```python
from build123d import *

# Parameters (mm, degrees)
SKETCH1_W           = 89
SKETCH1_H           = 57
BOSS_EXTRUDE1_DEPTH = 8
SKETCH2_W           = 32
SKETCH2_H           = 35.5
SKETCH2_H_2         = 6
SKETCH2_W_2         = 19
SKETCH2_H_3         = 1
CUT_EXTRUDE2_DEPTH  = 106.990565618
SKETCH3_R           = 2
CUT_EXTRUDE3_DEPTH  = 6.7


with BuildPart() as part:
    # Sketch1 → Boss-Extrude1 (new body)
    with BuildSketch(Plane(origin=(0, 0, 0), x_dir=(1, 0, 0), z_dir=(0, 1, 0))):
        with Locations((44.5, 28.5)):
            Rectangle(SKETCH1_W, SKETCH1_H)
    extrude(amount=BOSS_EXTRUDE1_DEPTH)

    # Sketch2 → Cut-Extrude2 (cut, through all)
    with BuildSketch(Plane(origin=(0, 8, 0), x_dir=(1, 0, 0), z_dir=(0, 1, 0))):
        with Locations((23.5, 28.25)):
            Rectangle(SKETCH2_W, SKETCH2_H)
        with Locations((23.5, 53)):
            Rectangle(SKETCH2_W, SKETCH2_H_2)
        with Locations((49, 53)):
            Rectangle(SKETCH2_W_2, SKETCH2_H_2)
        with Locations((49, 56.5)):
            Rectangle(SKETCH2_W_2, SKETCH2_H_3)
        with Locations((23.5, 56.5)):
            Rectangle(SKETCH2_W, SKETCH2_H_3)
    extrude(amount=-CUT_EXTRUDE2_DEPTH, mode=Mode.SUBTRACT)

    # Sketch3 → Cut-Extrude3 (cut)
    with BuildSketch(Plane.XY):
        with Locations((3.75, 4)):
            Circle(SKETCH3_R)
        with Locations((79, 4)):
            Circle(SKETCH3_R)
    cut_extrude3 = extrude(amount=-CUT_EXTRUDE3_DEPTH, mode=Mode.SUBTRACT)

    # Mirror1: Cut-Extrude3 across plane
    add(cut_extrude3.mirror(Plane.XY.offset(-28.5)), mode=Mode.SUBTRACT)


solid = part.part
```
The model under review builds one solid part; all positions refer to its coordinate system, in mm. A direction names the side the tool comes from. Round coordinates to 2 decimals unless told otherwise and drop trailing zeros. Loops run counter-clockwise (first coordinate to the right, second up) from the corner with the lowest first, then second, coordinate; pieces in that order, holes last. Notation, with made-up numbers: (70, 77) -> (87, 77) arc R21 ccw to (87, 105) -> close; hole circle Ø5 at (-18.75, 21.5). An arc over 180 degrees is marked (long way). Answer as a JSON object with one key per item and string values. Group by question number.
1) We need section D-D on x = 3.75. Write out the cut boundary in (y, z).
2) We need section B-B on z = -34. Write out the cut boundary in (x, y), then the cut area to 3 significant figures.
3) We need section C-C on y = 7. Write out the cut boundary in (x, z).
4) For line 1 (X direction, y = 4.5, z = -17.5); line 2 (Z direction, x = 13, y = 6.5); line 3 (Y direction, x = 3.75, z = -55.5), list the stretches that pass through material, from the lowest coordinate up. Write a range as [from, to].
5) We need section A-A on x = 32.5. Write out the cut boundary in (y, z).
6) For faces 1 (the face through (7.5, 4, -54)), 2 (the face through (7.5, 4, -28)), 3 (the face through (4, 4, -50.3)), list the 3-axis set-ups (+Z, -Z, +X, -X, +Y, -Y) from which the entire face can be reached by the end or side of a thin tool; tool diameter is ignored.
7) Mouldability with a two-part tool opening along X and no side actions: class faces 4 (the face through (54, 0, -29)), 5 (the face through (80.908, 4.601, -53.697)), 6 (the face through (89, 4, -28)), 7 (the face through (39.5, 4, -28)) as released by +X, released by -X, zero draft, split by the parting line, or undercut.
8) For pin 1 Ø3.5 at (x, y) = (79, 4) entering from -Z; pin 2 Ø2.5 at (x, y) = (43, 2.5) entering from -Z; pin 3 Ø2 at (x, z) = (38, -42) entering from +Y; pin 4 Ø1.2 at (x, y) = (78.5, 5) entering from +Z, all flat-tipped, find the tip position at first contact; note any pin that passes through.
Result set:
{
 "1": {"outline": "(0, -57) -> (2, -57) -> (2, -50.3) -> (6, -50.3) -> (6, -57) -> (8, -57) -> (8, 0) -> (6, 0) -> (6, -6.7) -> (2, -6.7) -> (2, 0) -> (0, 0) -> close"},
 "2": {"outline": "(0, 0) -> (7.5, 0) -> (7.5, 8) -> (0, 8) -> close; (39.5, 0) -> (89, 0) -> (89, 8) -> (39.5, 8) -> close", "area": "456 mm²"},
 "3": {"outline": "(0, -57) -> (7.5, -57) -> (7.5, -50) -> (58.5, -50) -> (58.5, -57) -> (89, -57) -> (89, 0) -> (0, 0) -> close; hole (7.5, -46) -> (39.5, -46) -> (39.5, -10.5) -> (7.5, -10.5) -> close"},
 "4": {"line 1": "[0, 7.5], [39.5, 89]", "line 2": "[-50, -46], [-10.5, 0]", "line 3": "[0, 2], [6, 8]"},
 "5": {"outline": "(0, -50) -> (8, -50) -> (8, -46) -> (0, -46) -> close; (0, -10.5) -> (8, -10.5) -> (8, 0) -> (0, 0) -> close"},
 "6": {"face 1": "-Z, +Y, -Y", "face 2": "+Y, -Y", "face 3": "-Z"},
 "7": {"face 4": "zero draft", "face 5": "undercut", "face 6": "released by +X", "face 7": "undercut"},
 "8": {"pin 1": "z = -50.3", "pin 2": "z = -50", "pin 3": "through", "pin 4": "z = -6.7"}
}
